Here's how the part is built. I have some questions about the finished solid (model axes, mm). Round coordinates to 2 decimals unless told otherwise and drop trailing zeros. Order: outer loops, then holes, each group sorted by start corner. A loop starts at its lowest first (then second) coordinate and runs counter-clockwise, first axis right, second up. Notation, with made-up numbers: (17, 65.5) -> (32, 65.5) arc R15 ccw to (32, 71.5) -> close; hole circle Ø8 at (18.5, -35.5). An arc over 180 degrees is marked (long way). Use a Markdown table: item, result. Add a question column.
(1) I want a section at B-B, the plane x = -16.5. Please give me the cut outline in (y, z).
(2) I want a section at A-A, the plane z = -17.5. Please give me the cut outline in (x, y), then the cut area to 3 significant figures.
(3) I'm going to push a flat-ended pin straight in: P1, Ø1.5, axis at x = -25, y = -1.5, coming from the +Z side. Where does the tip first touch, or does it pass through?
(4) If I drill on probe 1 along X at (y, z) = (-0.9, -24); probe 2 along X at (y, z) = (-1.95, 27.5); probe 3 along Z at (x, y) = (-26, -1.25), over which ranges is the centre line in solid material (lowest first)?
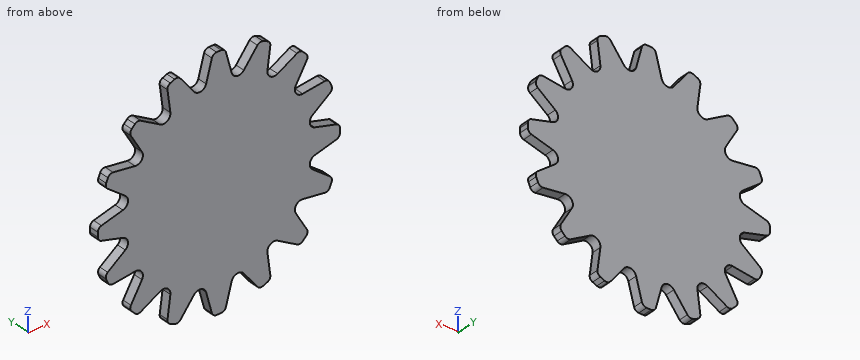
from build123d import *

# Parameters (mm, degrees)
F1_DEPTH = 2.54


with BuildPart() as f1:
    # F0 (on Front) → F1 (new body)
    with BuildSketch(Plane.XZ):
        with BuildLine():
            Line((0.612995, 31.75), (-0.612995, 31.75))
            ThreePointArc((-0.612995, 31.75), (-1.386122, 31.487559), (-1.839721, 30.8087))
            Line((-1.839721, 30.8087), (-3.348373, 25.178332))
            ThreePointArc((-3.348373, 25.178332), (-4.747603, 23.86781), (-6.541837, 24.543112))
            Line((-6.541837, 24.543112), (-10.090299, 29.167558))
            ThreePointArc((-10.090299, 29.167558), (-10.769158, 29.621157), (-11.583866, 29.567758))
            Line((-11.583866, 29.567758), (-12.716532, 29.098592))
            ThreePointArc((-12.716532, 29.098592), (-13.330377, 28.560265), (-13.489659, 27.759497))
            Line((-13.489659, 27.759497), (-12.728824, 21.980379))
            ThreePointArc((-12.728824, 21.980379), (-13.520029, 20.234153), (-15.436112, 20.171427))
            Line((-15.436112, 20.171427), (-20.484162, 23.08592))
            ThreePointArc((-20.484162, 23.08592), (-21.28493, 23.245202), (-22.017188, 22.884093))
            Line((-22.017188, 22.884093), (-22.884093, 22.017188))
            ThreePointArc((-22.884093, 22.017188), (-23.245202, 21.28493), (-23.08592, 20.484162))
            Line((-23.08592, 20.484162), (-20.171427, 15.436112))
            ThreePointArc((-20.171427, 15.436112), (-20.234153, 13.520029), (-21.980379, 12.728824))
            Line((-21.980379, 12.728824), (-27.759497, 13.489659))
            ThreePointArc((-27.759497, 13.489659), (-28.560265, 13.330377), (-29.098592, 12.716532))
            Line((-29.098592, 12.716532), (-29.567758, 11.583866))
            ThreePointArc((-29.567758, 11.583866), (-29.621157, 10.769158), (-29.167558, 10.090299))
            Line((-29.167558, 10.090299), (-24.543112, 6.541837))
            ThreePointArc((-24.543112, 6.541837), (-23.86781, 4.747603), (-25.178332, 3.348373))
            Line((-25.178332, 3.348373), (-30.8087, 1.839721))
            ThreePointArc((-30.8087, 1.839721), (-31.487559, 1.386122), (-31.75, 0.612995))
            Line((-31.75, 0.612995), (-31.75, -0.612995))
            ThreePointArc((-31.75, -0.612995), (-31.487559, -1.386122), (-30.8087, -1.839721))
            Line((-30.8087, -1.839721), (-25.178332, -3.348373))
            ThreePointArc((-25.178332, -3.348373), (-23.86781, -4.747603), (-24.543112, -6.541837))
            Line((-24.543112, -6.541837), (-29.167558, -10.090299))
            ThreePointArc((-29.167558, -10.090299), (-29.621157, -10.769158), (-29.567758, -11.583866))
            Line((-29.567758, -11.583866), (-29.098592, -12.716532))
            ThreePointArc((-29.098592, -12.716532), (-28.560265, -13.330377), (-27.759497, -13.489659))
            Line((-27.759497, -13.489659), (-21.980379, -12.728824))
            ThreePointArc((-21.980379, -12.728824), (-20.234153, -13.520029), (-20.171427, -15.436112))
            Line((-20.171427, -15.436112), (-23.08592, -20.484162))
            ThreePointArc((-23.08592, -20.484162), (-23.245202, -21.28493), (-22.884093, -22.017188))
            Line((-22.884093, -22.017188), (-22.017188, -22.884093))
            ThreePointArc((-22.017188, -22.884093), (-21.28493, -23.245202), (-20.484162, -23.08592))
            Line((-20.484162, -23.08592), (-15.436112, -20.171427))
            ThreePointArc((-15.436112, -20.171427), (-13.520029, -20.234153), (-12.728824, -21.980379))
            Line((-12.728824, -21.980379), (-13.489659, -27.759497))
            ThreePointArc((-13.489659, -27.759497), (-13.330377, -28.560265), (-12.716532, -29.098592))
            Line((-12.716532, -29.098592), (-11.583866, -29.567758))
            ThreePointArc((-11.583866, -29.567758), (-10.769158, -29.621157), (-10.090299, -29.167558))
            Line((-10.090299, -29.167558), (-6.541837, -24.543112))
            ThreePointArc((-6.541837, -24.543112), (-4.747603, -23.86781), (-3.348373, -25.178332))
            Line((-3.348373, -25.178332), (-1.839721, -30.8087))
            ThreePointArc((-1.839721, -30.8087), (-1.386122, -31.487559), (-0.612995, -31.75))
            Line((-0.612995, -31.75), (0.612995, -31.75))
            ThreePointArc((0.612995, -31.75), (1.386122, -31.487559), (1.839721, -30.8087))
            Line((1.839721, -30.8087), (3.348373, -25.178332))
            ThreePointArc((3.348373, -25.178332), (4.747603, -23.86781), (6.541837, -24.543112))
            Line((6.541837, -24.543112), (10.090299, -29.167558))
            ThreePointArc((10.090299, -29.167558), (10.769158, -29.621157), (11.583866, -29.567758))
            Line((11.583866, -29.567758), (12.716532, -29.098592))
            ThreePointArc((12.716532, -29.098592), (13.330377, -28.560265), (13.489659, -27.759497))
            Line((13.489659, -27.759497), (12.728824, -21.980379))
            ThreePointArc((12.728824, -21.980379), (13.520029, -20.234153), (15.436112, -20.171427))
            Line((15.436112, -20.171427), (20.484162, -23.08592))
            ThreePointArc((20.484162, -23.08592), (21.28493, -23.245202), (22.017188, -22.884093))
            Line((22.017188, -22.884093), (22.884093, -22.017188))
            ThreePointArc((22.884093, -22.017188), (23.245202, -21.28493), (23.08592, -20.484162))
            Line((23.08592, -20.484162), (20.171427, -15.436112))
            ThreePointArc((20.171427, -15.436112), (20.234153, -13.520029), (21.980379, -12.728824))
            Line((21.980379, -12.728824), (27.759497, -13.489659))
            ThreePointArc((27.759497, -13.489659), (28.560265, -13.330377), (29.098592, -12.716532))
            Line((29.098592, -12.716532), (29.567758, -11.583866))
            ThreePointArc((29.567758, -11.583866), (29.621157, -10.769158), (29.167558, -10.090299))
            Line((29.167558, -10.090299), (24.543112, -6.541837))
            ThreePointArc((24.543112, -6.541837), (23.86781, -4.747603), (25.178332, -3.348373))
            Line((25.178332, -3.348373), (30.8087, -1.839721))
            ThreePointArc((30.8087, -1.839721), (31.487559, -1.386122), (31.75, -0.612995))
            Line((31.75, -0.612995), (31.75, 0.612995))
            ThreePointArc((31.75, 0.612995), (31.487559, 1.386122), (30.8087, 1.839721))
            Line((30.8087, 1.839721), (25.178332, 3.348373))
            ThreePointArc((25.178332, 3.348373), (23.86781, 4.747603), (24.543112, 6.541837))
            Line((24.543112, 6.541837), (29.167558, 10.090299))
            ThreePointArc((29.167558, 10.090299), (29.621157, 10.769158), (29.567758, 11.583866))
            Line((29.567758, 11.583866), (29.098592, 12.716532))
            ThreePointArc((29.098592, 12.716532), (28.560265, 13.330377), (27.759497, 13.489659))
            Line((27.759497, 13.489659), (21.980379, 12.728824))
            ThreePointArc((21.980379, 12.728824), (20.234153, 13.520029), (20.171427, 15.436112))
            Line((20.171427, 15.436112), (23.08592, 20.484162))
            ThreePointArc((23.08592, 20.484162), (23.245202, 21.28493), (22.884093, 22.017188))
            Line((22.884093, 22.017188), (22.017188, 22.884093))
            ThreePointArc((22.017188, 22.884093), (21.28493, 23.245202), (20.484162, 23.08592))
            Line((20.484162, 23.08592), (15.436112, 20.171427))
            ThreePointArc((15.436112, 20.171427), (13.520029, 20.234153), (12.728824, 21.980379))
            Line((12.728824, 21.980379), (13.489659, 27.759497))
            ThreePointArc((13.489659, 27.759497), (13.330377, 28.560265), (12.716532, 29.098592))
            Line((12.716532, 29.098592), (11.583866, 29.567758))
            ThreePointArc((11.583866, 29.567758), (10.769158, 29.621157), (10.090299, 29.167558))
            Line((10.090299, 29.167558), (6.541837, 24.543112))
            ThreePointArc((6.541837, 24.543112), (4.747603, 23.86781), (3.348373, 25.178332))
            Line((3.348373, 25.178332), (1.839721, 30.8087))
            ThreePointArc((1.839721, 30.8087), (1.386122, 31.487559), (0.612995, 31.75))
        make_face()
    extrude(amount=F1_DEPTH)


solid = f1.part
Taken from the geometry:
| question | item | result |
|---|---|---|
| 1 | outline | (-2.54, -20.79) -> (0, -20.79) -> (0, 20.79) -> (-2.54, 20.79) -> close |
| 2 | outline | (-21.36, -2.54) -> (21.36, -2.54) -> (21.36, 0) -> (-21.36, 0) -> close |
| 2 | area | 109 mm2 |
| 3 | P1 | stops at z = 13.23 |
| 4 | probe 1 | x = -12.99 to -5.86, -4.34 to 4.34, 5.86 to 12.99 |
| 4 | probe 2 | x = -13.46 to -8.81, -2.73 to 2.73, 8.81 to 13.46 |
| 4 | probe 3 | z = -13.26 to -7.66, -3.13 to 3.13, 7.66 to 13.26 |
